Check sheet for the modelled part. Datum: model origin and axes. Units: mm. A direction names the side the tool comes from. Coordinates: 2 decimals unless noted, no trailing zeros. Order: outer loops, then holes, each group sorted by start corner. A loop starts at its lowest first (then second) coordinate and runs counter-clockwise, first axis right, second up.
from build123d import *

# Parameters (mm, degrees)
SKETCH_1_R             = 4.25
SKETCH_1_R_2           = 1.55
EXTRUDE_1_DEPTH        = 2
FILLET_1_R             = 1
EXTRUDE_2_DEPTH        = 4
SKETCH_3_R             = 0.75
CUT_EXTRUDE_1_DEPTH    = 5
FILLET_2_R             = 1
FILLET_2_OF_MIRROR_1_R = 1
CUT_EXTRUDE_2_DEPTH    = 5
FILLET_3_R             = 1


with BuildPart() as part:
    # 草图1 → 凸台-拉伸1 (new body, symmetric)
    with BuildSketch(Plane.XY):
        with BuildLine():
            Line((-17.997731807, 4.466704665), (-2.130665002, 16.641933245))
            ThreePointArc((-2.130665002, 16.641933245), (0, 17.365196554), (2.130665002, 16.641933245))
            Line((2.130665002, 16.641933245), (17.997731807, 4.466704665))
            ThreePointArc((17.997731807, 4.466704665), (17.415077222, -1.449086621), (12.367066806, 1.689967974))
            Line((12.367066806, 1.689967974), (8.585249457, 1.689967974))
            ThreePointArc((8.585249457, 1.689967974), (0, -8.75), (-8.585249457, 1.689967974))
            Line((-8.585249457, 1.689967974), (-12.367066806, 1.689967974))
            ThreePointArc((-12.367066806, 1.689967974), (-17.415077222, -1.449086621), (-17.997731807, 4.466704665))
        make_face()
        Circle(SKETCH_1_R, mode=Mode.SUBTRACT)
        with Locations((-15.867066806, 1.689967974)):
            Circle(SKETCH_1_R_2, mode=Mode.SUBTRACT)
        with Locations((0, 13.865196554)):
            Circle(SKETCH_1_R_2, mode=Mode.SUBTRACT)
        with Locations((15.867066806, 1.689967974)):
            Circle(SKETCH_1_R_2, mode=Mode.SUBTRACT)
    extrude(amount=EXTRUDE_1_DEPTH, both=True)

    # 圆角1
    fillet_1_edges = [part.edges().sort_by_distance(p)[0] for p in [
        (12.367066806, 1.689967974, 0),
        (8.585249457, 1.689967974, 0),
        (-8.585249457, 1.689967974, 0),
        (-12.367066806, 1.689967974, 0),
    ]]
    fillet(fillet_1_edges, radius=FILLET_1_R)

    # 草图2 → 凸台-拉伸2 (add)
    with BuildSketch(Plane.XY.offset(2)):
        with BuildLine():
            Line((-18.971604722, 0.073847828), (-22.953372788, 7.722753116))
            Line((-22.953372788, 7.722753116), (-8.084856844, 19.131766671))
            Line((-8.084856844, 19.131766671), (-3.978157764, 19.131766671))
            Line((-3.978157764, 19.131766671), (-19.924559904, 6.895661948))
            Line((-19.924559904, 6.895661948), (-18.037399474, 4.436266594))
            Line((-18.037399474, 4.436266594), (-17.997731807, 4.466704665))
            ThreePointArc((-17.997731807, 4.466704665), (-19.284102831, 2.447506623), (-18.971604722, 0.073847828))
        make_face()
    extrude_2 = extrude(amount=-EXTRUDE_2_DEPTH)

    # 草图3 → 切除-拉伸1 (cut, through all)
    with BuildSketch(Plane.XY.offset(2)):
        with Locations((-19.329544899, 7.35223302)):
            Circle(SKETCH_3_R)
        with Locations((-17.442384469, 4.892837665)):
            Circle(SKETCH_3_R)
    cut_extrude_1 = extrude(amount=-CUT_EXTRUDE_1_DEPTH, mode=Mode.SUBTRACT)

    # 圆角2
    fillet_2_edges = [part.edges().sort_by_distance(p)[0] for p in [
        (-22.953372788, 7.722753116, 0),
        (-8.084856844, 19.131766671, 0),
        (-3.978157764, 19.131766671, 0),
    ]]
    fillet(fillet_2_edges, radius=FILLET_2_R)

    # 镜向1: 凸台-拉伸2, 切除-拉伸1 across plane
    add(extrude_2.mirror(Plane(origin=(0, 0, 0), x_dir=(0, 0, 1), z_dir=(1, 0, 0))))
    add(cut_extrude_1.mirror(Plane(origin=(0, 0, 0), x_dir=(0, 0, 1), z_dir=(1, 0, 0))), mode=Mode.SUBTRACT)

    # 圆角2 of 镜向1
    fillet_2_of_mirror_1_edges = [part.edges().sort_by_distance(p)[0] for p in [
        (22.953372788, 7.722753116, 0),
        (8.084856844, 19.131766671, 0),
        (3.978157764, 19.131766671, 0),
    ]]
    fillet(fillet_2_of_mirror_1_edges, radius=FILLET_2_OF_MIRROR_1_R)

    # 草图4 → 切除-拉伸2 (cut, through all)
    with BuildSketch(Plane.XY.offset(2)):
        with BuildLine():
            Line((-12.778730503, 4.689967974), (-3.052637302, 12.153061775))
            ThreePointArc((-3.052637302, 12.153061775), (0, 10.365196554), (3.052637302, 12.153061775))
            Line((3.052637302, 12.153061775), (12.778730503, 4.689967974))
            Line((12.778730503, 4.689967974), (7.38692767, 4.689967974))
            ThreePointArc((7.38692767, 4.689967974), (0, 8.75), (-7.38692767, 4.689967974))
            Line((-7.38692767, 4.689967974), (-12.778730503, 4.689967974))
        make_face()
    extrude(amount=-CUT_EXTRUDE_2_DEPTH, mode=Mode.SUBTRACT)

    # 圆角3
    fillet_3_edges = [part.edges().sort_by_distance(p)[0] for p in [
        (-7.38692767, 4.689967974, 0),
        (-12.778730503, 4.689967974, 0),
        (-3.052637302, 12.153061775, 0),
        (3.052637302, 12.153061775, 0),
        (12.778730503, 4.689967974, 0),
        (7.38692767, 4.689967974, 0),
    ]]
    fillet(fillet_3_edges, radius=FILLET_3_R)


solid = part.part
(1) Go/stop test with flat-tipped pins: P1, Ø0.9, axis at x = 10.5, z = -0.5, coming from the -Y side; P2, Ø0.6, axis at x = 9, z = 0, coming from the +Y side; P3, Ø1, axis at y = -3.5, z = 1, coming from the -X side. Record where each tip stops, or that it passes through.
Filled in:
P1: stops at y = 1.69
P2: stops at y = 18.66
P3: stops at x = -8.22
(2) Cross-section at D-D (z = -0.5). Count the separate pieces of the cut face and the enclosed holes in it, and give its area (3 significant figures).
Filled in:
separate pieces: 1
enclosed holes: 5
area: 513 mm2
(3) Cross-section at A-A (x = 0). Enter the section's corners in (y, z), and give its area (3 significant figures).
Filled in:
outline: (-8.75, -2) - (-4.25, -2) - (-4.25, 2) - (-8.75, 2) - close; (4.25, -2) - (8.75, -2) - (8.75, 2) - (4.25, 2) - close; (10.37, -2) - (12.32, -2) - (12.32, 2) - (10.37, 2) - close; (15.42, -2) - (17.37, -2) - (17.37, 2) - (15.42, 2) - close
area: 51.6 mm2
(4) Cross-section at B-B (y = 6). Enter the section's corners in (x, z).
Filled in:
outline: (-22.06, -2) - (-19.24, -2) - (-19.24, 2) - (-22.06, 2) - close; (-16, -2) - (-10.78, -2) - (-10.78, 2) - (-16, 2) - close; (-6.37, -2) - (6.37, -2) - (6.37, 2) - (-6.37, 2) - close; (10.78, -2) - (16, -2) - (16, 2) - (10.78, 2) - close; (19.24, -2) - (22.06, -2) - (22.06, 2) - (19.24, 2) - close
(5) Release check for a two-part mould opening along X. For faces 3 (the cylindrical face through (-22.657, 7.647, -0.028)), 4 (the flat face through (20.744, 3.478, 0.028)), 5 (the flat face through (-9.59, 10.92, 0.03)) record: +X half, -X half, draft (parallel to the pull), parting line (faces both ways), or undercut.
Filled in:
face 3: -X half
face 4: +X half
face 5: undercut
(6) Thickness scan on probe 1 along X at (y, z) = (7.25, 1.85); probe 2 along X at (y, z) = (16.5, 1.45); probe 3 along X at (y, z) = (17, 1.45). Record the ranges inside material, lowest first.
Filled in:
probe 1: x = -22.66 to -20.07, -14.37 to -9.44, -4.9 to 4.9, 9.44 to 14.37, 20.07 to 22.66
probe 2: x = -11.51 to -7.41, -2.32 to 2.32, 7.41 to 11.51
probe 3: x = -10.86 to -6.76, -1.56 to 1.56, 6.76 to 10.86
(7) Tool access check on faces 1 (the cylindrical face through (15.48, -1.79, 0.03)), 2 (the cylindrical face through (-5.972, 18.437, -0.028)). Record the directions out of +Z, -Z, +X, -X, +Y, -Y that give a thin tool (end or side, any length) a straight path to the whole face; none if there is none.
Filled in:
face 1: +Z, -Z, -Y
face 2: +Z, -Z
(8) Cross-section at C-C (y = -2.5). Enter the section's corners in (x, z).
Filled in:
outline: (-8.39, -2) - (-3.44, -2) - (-3.44, 2) - (-8.39, 2) - close; (3.44, -2) - (8.39, -2) - (8.39, 2) - (3.44, 2) - close
